Here's the drawing with two shaded views (mm, measured from the low corner). I have some questions. Round coordinates to 2 decimals unless told otherwise and drop trailing zeros. Loops run counter-clockwise (first coordinate to the right, second up) from the corner with the lowest first, then second, coordinate; pieces in that order, holes last.
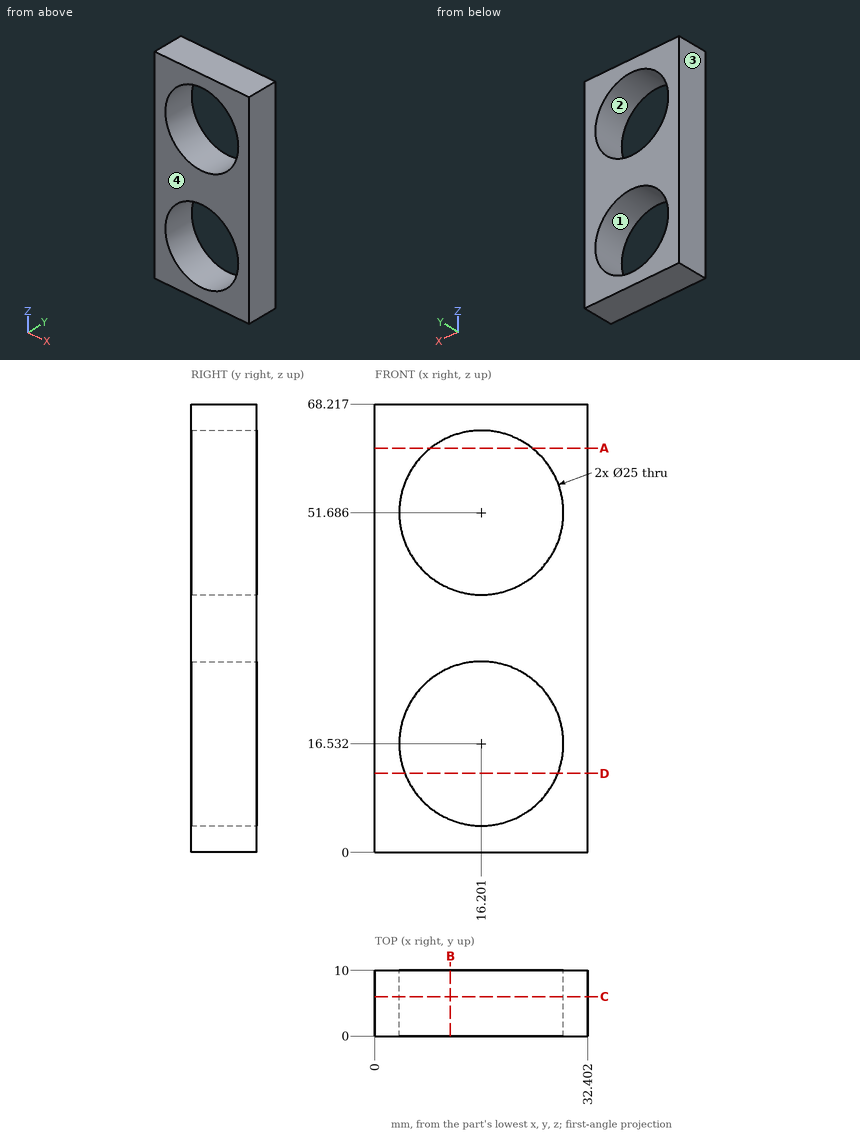
Item 1: If I drill on line 1 along Z through (x, y) = (23, 8.25) (1 decimal); line 2 along Z through (x, y) = (14.5, 3.75) (1 decimal); line 3 along X through (y, z) = (7.75, 52) (1 decimal), over which ranges is the centre line in solid material (lowest first)?
Results list:
line 1: z = 0 to 6, 27 to 41.2, 62.2 to 68.2
line 2: z = 0 to 4.1, 28.9 to 39.3, 64.1 to 68.2
line 3: x = 0 to 3.7, 28.7 to 32.4
Item 2: If we section it at C-C, the plane y = 6: Please give me the cut outline in (x, z) (1 decimal).
Results list:
outline: (0, 0) - (32.4, 0) - (32.4, 68.2) - (0, 68.2) - close; hole circle Ø25 at (16.2, 16.5); hole circle Ø25 at (16.2, 51.7)
Item 3: If we section it at A-A, the plane z = 61.5: Please give me the cut outline in (x, y).
Results list:
outline: (0, 0) - (8.46, 0) - (8.46, 10) - (0, 10) - close; (23.94, 0) - (32.4, 0) - (32.4, 10) - (23.94, 10) - close
Item 4: If we section it at D-D, the plane z = 12: Please give me the cut outline in (x, y).
Results list:
outline: (0, 0) - (4.55, 0) - (4.55, 10) - (0, 10) - close; (27.85, 0) - (32.4, 0) - (32.4, 10) - (27.85, 10) - close
Item 5: If we section it at B-B, the plane x = 11.5: Count the separate pieces of the cut face and the enclosed holes in it, then the cut area to 3 significant figures.
Results list:
separate pieces: 3
enclosed holes: 0
area: 219 mm2
Item 6: We'd pull the mould along X, two halves only. Please class the marked faces 1, 2, 3 and 4: released by +X, released by -X, zero draft, split by the parting line, or undercut.
Results list:
face 1: undercut
face 2: undercut
face 3: released by -X
face 4: zero draft
